Check sheet for the drawn part. Datum: minimum x, y, z corner. Units: mm. A direction names the side the tool comes from. Coordinates: 2 decimals unless noted, no trailing zeros. Write each loop counter-clockwise with the first axis right and the second up, starting at its lowest first coordinate (ties: lowest second). Pieces come first, ordered by that corner, then holes. Notation, with made-up numbers: M 24.25,81 L 29.25,81 A7 cw 29.25,89 Z; hole C 82.5,12.25 d6. An arc over 180 degrees is marked long. Answer as a JSON object with one key per item and string values. Group by question number.
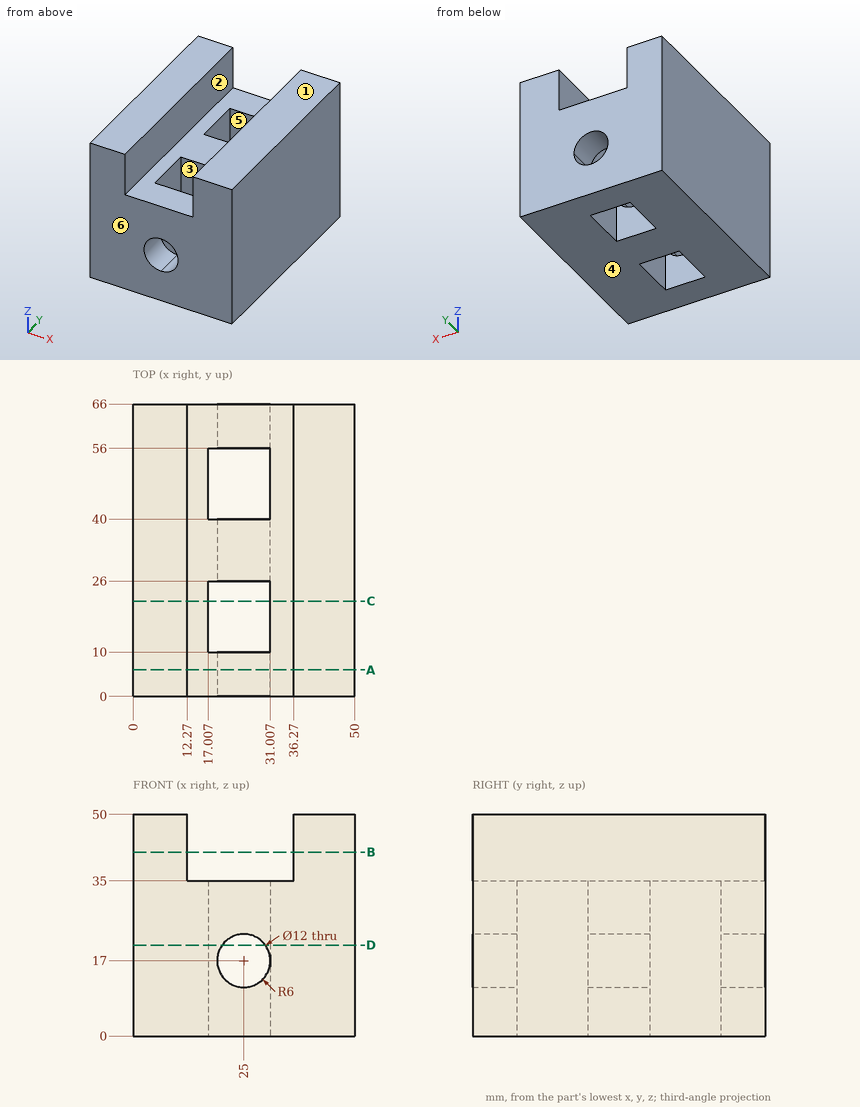
1) Section check D-D (z = 20.5). Record the cut outline in (x, y), then the cut area to 3 significant figures.
2) Material ranges on probe 1 along Y at (x, z) = (23, 3.5); probe 2 along X at (y, z) = (34.5, 17); probe 3 along X at (y, z) = (17, 13.5), recorded low to high. Write a range as [from, to].
3) Section check B-B (z = 41.5). Record the cut outline in (x, y).
4) Draft check along Y on the marked faces 4, 5 and 6. Enter one of: +Y half, -Y half, draft (parallel to the pull), parting line (faces both ways), or undercut.
5) Go/stop test with a flat-tipped pin: pin 1 Ø1 at (y, z) = (10, 11) entering from -X. Record where the tip stops, or that it passes through.
6) Section check A-A (y = 6). Record the cut outline in (x, z), then the cut area to 3 significant figures.
7) Set-up check for the marked faces 1, 2 and 3: record each of +Z, -Z, +X, -X, +Y, -Y from which the full face is reachable in a straight line by a thin tool's end or side.
8) Section check C-C (y = 21.5). Record the cut outline in (x, z).
Entries:
{
 "1": {"outline": "M 0,0 L 20.13,0 L 20.13,10 L 17.01,10 L 17.01,26 L 20.13,26 L 20.13,40 L 17.01,40 L 17.01,56 L 20.13,56 L 20.13,66 L 0,66 Z; M 29.87,0 L 50,0 L 50,66 L 29.87,66 L 29.87,56 L 31.01,56 L 31.01,40 L 29.87,40 L 29.87,26 L 31.01,26 L 31.01,10 L 29.87,10 Z", "area": "2,520 mm^2"},
 "2": {"probe 1": "[0, 10], [26, 40], [56, 66]", "probe 2": "[0, 19], [31, 50]", "probe 3": "[0, 17.01], [31.01, 50]"},
 "3": {"outline": "M 0,0 L 12.27,0 L 12.27,66 L 0,66 Z; M 36.27,0 L 50,0 L 50,66 L 36.27,66 Z"},
 "4": {"face 4": "draft", "face 5": "undercut", "face 6": "-Y half"},
 "5": {"pin 1": "x = 0"},
 "6": {"outline": "M 0,0 L 50,0 L 50,50 L 36.27,50 L 36.27,35 L 12.27,35 L 12.27,50 L 0,50 Z; hole M 25,11 A6 ccw 31,17 A6 ccw long Z", "area": "2,030 mm^2"},
 "7": {"face 1": "+Z, +X, -X, +Y, -Y", "face 2": "+Z, +Y, -Y", "face 3": "+Z, -Z"},
 "8": {"outline": "M 0,0 L 17.01,0 L 17.01,35 L 12.27,35 L 12.27,50 L 0,50 Z; M 31.01,0 L 50,0 L 50,50 L 36.27,50 L 36.27,35 L 31.01,35 Z"}
}
